Verification items for this drawing (mm, ordinates from the low corner). A direction names the side the tool comes from. Round coordinates to 2 decimals unless told otherwise and drop trailing zeros. Loops run counter-clockwise (first coordinate to the right, second up) from the corner with the lowest first, then second, coordinate; pieces in that order, holes last. Notation, with made-up numbers: (26.5, -30) - (51.5, -30) arc R11 ccw to (51.5, -17) - close; hole circle Ø2 at (74.25, 20.5). An arc over 180 degrees is marked (long way). Use a Markdown table: item, result. Add a question column.
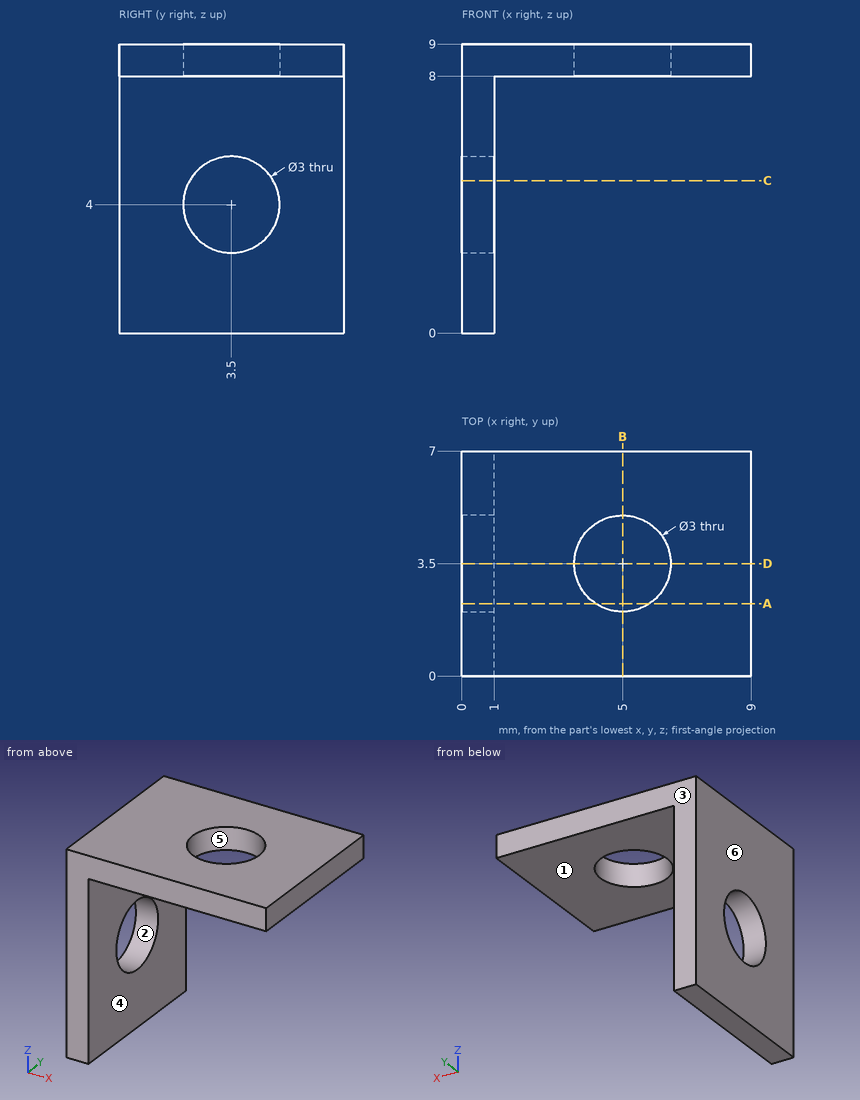
Q1. Release check for a two-part mould opening along X. For the marked faces 3, 4, 5 and 6 record: +X half, -X half, draft (parallel to the pull), parting line (faces both ways), or undercut.
Q2. Section check D-D on y = 3.5. Record the cut outline in (x, z), plus the area to 3 significant figures.
Q3. Section check B-B on x = 5. Record the cut outline in (y, z).
Q4. Set-up check for the marked faces 1 and 2: record each of +Z, -Z, +X, -X, +Y, -Y from which the full face is reachable in a straight line by a thin tool's end or side.
Q5. Section check C-C on z = 4.75. Record the cut outline in (x, y).
Q6. Thickness scan on line 1 along Z through (x, y) = (0.5, 3.5); line 2 along Z through (x, y) = (2, 3.75); line 3 along X through (y, z) = (2.25, 2.75). Record the ranges inside material, lowest first.
Q7. Go/stop test with flat-tipped pins: pin 1 Ø3.5 at (y, z) = (3.5, 4.5) entering from +X; pin 2 Ø4 at (x, y) = (1, 3.5) entering from -Z. Record where each tip stops, or that it passes through.
Q8. Section check A-A on y = 2.25. Record the cut outline in (x, z), plus the area to 3 significant figures.
Determined:
| question | item | result |
|---|---|---|
| 1 | face 3 | draft |
| 1 | face 4 | +X half |
| 1 | face 5 | undercut |
| 1 | face 6 | -X half |
| 2 | outline | (0, 0) - (1, 0) - (1, 2.5) - (0, 2.5) - close; (0, 5.5) - (1, 5.5) - (1, 8) - (3.5, 8) - (3.5, 9) - (0, 9) - close; (6.5, 8) - (9, 8) - (9, 9) - (6.5, 9) - close |
| 2 | area | 11.0 mm² |
| 3 | outline | (0, 8) - (2, 8) - (2, 9) - (0, 9) - close; (5, 8) - (7, 8) - (7, 9) - (5, 9) - close |
| 4 | face 1 | -Z, +X, +Y, -Y |
| 4 | face 2 | +X, -X |
| 5 | outline | (0, 0) - (1, 0) - (1, 2.2) - (0, 2.2) - close; (0, 4.8) - (1, 4.8) - (1, 7) - (0, 7) - close |
| 6 | line 1 | z = 0 to 2.5, 5.5 to 9 |
| 6 | line 2 | z = 8 to 9 |
| 6 | line 3 | x = 0 to 1 |
| 7 | pin 1 | stops at x = 1 |
| 7 | pin 2 | stops at z = 0 |
| 8 | outline | (0, 0) - (1, 0) - (1, 3.17) - (0, 3.17) - close; (0, 4.83) - (1, 4.83) - (1, 8) - (4.17, 8) - (4.17, 9) - (0, 9) - close; (5.83, 8) - (9, 8) - (9, 9) - (5.83, 9) - close |
| 8 | area | 13.7 mm² |
